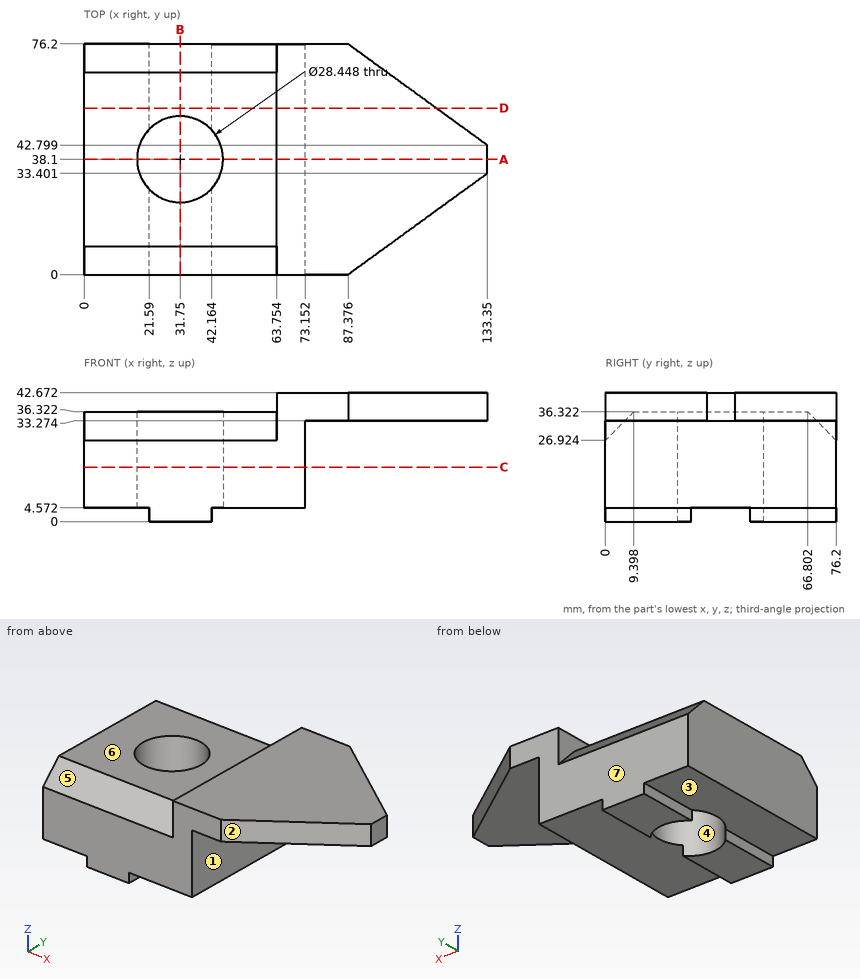
The drawing under review shows one solid part. Ordinate dimensions are in mm from its lowest x, y, z. A direction names the side the tool comes from. Round coordinates to 2 decimals unless told otherwise and drop trailing zeros. Loops run counter-clockwise (first coordinate to the right, second up) from the corner with the lowest first, then second, coordinate; pieces in that order, holes last. Notation, with made-up numbers: (4.25, 5) - (18.25, 5) arc R16 cw to (18.25, 30) - close; hole circle Ø8 at (28, 42). An arc over 180 degrees is marked (long way). Use one line per item in the form item = value.
Item 1: For line 1 (Y direction, x = 31.75, z = 22.5); line 2 (X direction, y = 38, z = 18); line 3 (Z direction, x = 93.5, y = 60), list the stretches that pass through material, from the lowest coordinate up.
Answers:
line_1 = 0 to 23.88, 52.32 to 76.2
line_2 = 0 to 17.53, 45.97 to 73.15
line_3 = 33.27 to 42.67
Item 2: Mouldability with a two-part tool opening along Y and no side actions: class the marked faces 4, 5, 6 and 7 as +Y half, -Y half, draft (parallel to the pull), parting line (faces both ways), or undercut.
Answers:
face_4 = undercut
face_5 = -Y half
face_6 = draft
face_7 = +Y half
Item 3: Consider section C-C on z = 18. Write out the cut boundary in (x, y).
Answers:
outline = (0, 0) - (73.15, 0) - (73.15, 76.2) - (0, 76.2) - close; hole circle Ø28.45 at (31.75, 38.1)
Item 4: Tool access review of the marked faces 1, 2 and 3: name each direction out of +Z, -Z, +X, -X, +Y, -Y from which nothing blocks a thin tool from reaching the whole face with its end or side.
Answers:
face_1 = -Z, +X, +Y, -Y
face_2 = +Z, -Z, +X, -Y
face_3 = -Z, -X, +Y, -Y
Item 5: Consider section B-B on x = 31.75. Write out the cut boundary in (y, z), then the cut area to 3 significant figures.
Answers:
outline = (0, 0) - (23.88, 0) - (23.88, 36.32) - (9.4, 36.32) - (0, 26.92) - close; (52.32, 0) - (76.2, 0) - (76.2, 26.92) - (66.8, 36.32) - (52.32, 36.32) - close
area = 1,650 mm^2
Item 6: Consider section D-D on y = 55. Write out the cut boundary in (x, z).
Answers:
outline = (0, 4.57) - (21.59, 4.57) - (21.59, 0) - (42.16, 0) - (42.16, 4.57) - (73.15, 4.57) - (73.15, 33.27) - (116.56, 33.27) - (116.56, 42.67) - (63.75, 42.67) - (63.75, 36.32) - (0, 36.32) - close
Item 7: Clearance check with flat-ended pins moving along their axes: P1, Ø5, axis at y = 57.5, z = 3.5, coming from the +X side; P2, Ø8, axis at x = 93, y = 39.5, coming from the -Z side; P3, Ø17, axis at x = 41.5, y = 42.5, coming from the +Z side. State where each tip first meets the part, or that it passes through.
Answers:
P1 = 73.15
P2 = 33.27
P3 = 36.32
Item 8: Consider section A-A on y = 38.1. Write out the cut boundary in (x, z).
Answers:
outline = (0, 4.57) - (17.53, 4.57) - (17.53, 36.32) - (0, 36.32) - close; (45.97, 4.57) - (73.15, 4.57) - (73.15, 33.27) - (133.35, 33.27) - (133.35, 42.67) - (63.75, 42.67) - (63.75, 36.32) - (45.97, 36.32) - close
